from build123d import *

# Parameters (mm, degrees)
SKETCH1_W           = 1280
SKETCH1_H           = 1140
BOSS_EXTRUDE1_DEPTH = 40
SKETCH2_W           = 40
SKETCH2_H           = 1140
BOSS_EXTRUDE2_DEPTH = 80
SKETCH3_W           = 1200
SKETCH3_H           = 40
BOSS_EXTRUDE3_DEPTH = 80


with BuildPart() as part:
    # Sketch1 → Boss-Extrude1 (new body)
    with BuildSketch(Plane(origin=(0, 0, 0), x_dir=(1, 0, 0), z_dir=(0, 1, 0))):
        with Locations((640, -570)):
            Rectangle(SKETCH1_W, SKETCH1_H)
    extrude(amount=BOSS_EXTRUDE1_DEPTH)

    # Sketch2 → Boss-Extrude2 (add)
    with BuildSketch(Plane(origin=(0, 40, 0), x_dir=(1, 0, 0), z_dir=(0, 1, 0))):
        with Locations((1260, -570)):
            Rectangle(SKETCH2_W, SKETCH2_H)
        with Locations((20, -570)):
            Rectangle(SKETCH2_W, SKETCH2_H)
    extrude(amount=BOSS_EXTRUDE2_DEPTH)

    # Sketch3 → Boss-Extrude3 (add)
    with BuildSketch(Plane(origin=(0, 40, 0), x_dir=(1, 0, 0), z_dir=(0, 1, 0))):
        with Locations((640, -20)):
            Rectangle(SKETCH3_W, SKETCH3_H)
    extrude(amount=BOSS_EXTRUDE3_DEPTH)


solid = part.part
Read the model definition and answer for the solid it produces. Units are mm, in the model's axes. A direction names the side the tool comes from. Round coordinates to 2 decimals unless told otherwise and drop trailing zeros. Order: outer loops, then holes, each group sorted by start corner. A loop starts at its lowest first (then second) coordinate and runs counter-clockwise, first axis right, second up.
1) Flat-ended cylindrical pins translate along their axes: pin 1 (2 mm diameter, centred on y = 40.5, z = 278.5, fed in from -X); pin 2 (4 mm diameter, centred on x = 618, z = 620.5, fed in from +Y); pin 3 (10 mm diameter, centred on x = 552, y = 71.5, fed in from +Z). Find the tip coordinate at first contact, or state that the pin passes through.
2) The part is cut by section C-C on x = 263. Write down the section's boundary in (y, z), plus the area to 3 significant figures.
3) The part is cut by section A-A on y = 74.5. Write down the section's boundary in (x, z).
4) Straight lines are drawn through the part: L1, parallel to X at y = 82, z = 1060.5; L2, parallel to Z at x = 182.5, y = 92. For each, find the intervals that lie inside material, in ascending order.
5) The part is cut by section B-B on z = 893. Write down the section's boundary in (x, y).
6) For faces 4 (the face through (1240, 79, 598)), 5 (the face through (631, 59, 0)), determine the directions among +Z, -Z, +X, -X, +Y, -Y from which every point of the face is accessible in a straight line to the end or side of a thin tool.
7) The mould has two halves that part along X. Classify faces 1 (the face through (0, 59, 578)), 2 (the face through (637, 120, 18)), 3 (the face through (632, 40, 582)): released by +X, released by -X, zero draft, split by the parting line, or undercut.
Resolved:
1. pin 1: stops at x = 0
1. pin 2: stops at y = 40
1. pin 3: stops at z = 40
2. outline: (0, 0) - (120, 0) - (120, 40) - (40, 40) - (40, 1140) - (0, 1140) - close
2. area: 48,800 mm2
3. outline: (0, 0) - (1280, 0) - (1280, 1140) - (1240, 1140) - (1240, 40) - (40, 40) - (40, 1140) - (0, 1140) - close
4. L1: x = 0 to 40, 1240 to 1280
4. L2: z = 0 to 40
5. outline: (0, 0) - (1280, 0) - (1280, 120) - (1240, 120) - (1240, 40) - (40, 40) - (40, 120) - (0, 120) - close
6. face 4: +Z, +Y
6. face 5: -Z, +X, -X, +Y, -Y
7. face 1: released by -X
7. face 2: zero draft
7. face 3: undercut
